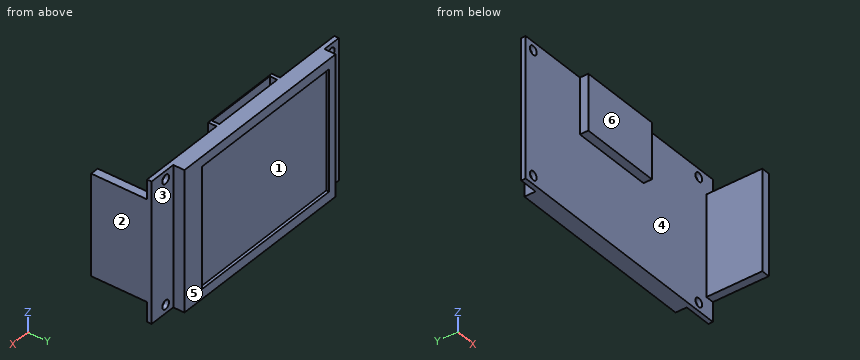
```python
from build123d import *

# Parameters (mm, degrees)
SKETCH1_W          = 86.3
SKETCH1_H          = 50.1
CIRCUIT_DEPTH      = 1.6
SKETCH2_R          = 1.57
SCREW_HOLES_DEPTH  = 50.919785657
SKETCH3_W          = 69.7
SKETCH3_H          = 50.1
LCD_DEPTH          = 4
SKETCH4_W          = 3
SKETCH4_H          = 36.1
PINS_DEPTH         = 20
SKETCH6_W          = 29.3
SKETCH6_H          = 20
SD_SLOT_DEPTH      = 3
SKETCH8_W          = 26.7
SKETCH8_H          = 2.65
CUT_EXTRUDE2_DEPTH = 5
SKETCH9_W          = 58.7
SKETCH9_H          = 43.1
CUT_EXTRUDE3_DEPTH = 1


with BuildPart() as part:
    # Sketch1 → CIRCUIT (new body)
    with BuildSketch(Plane(origin=(0, 0, 0), x_dir=(1, 0, 0), z_dir=(0, 1, 0))):
        Rectangle(SKETCH1_W, SKETCH1_H)
    extrude(amount=CIRCUIT_DEPTH)

    # Sketch2 → SCREW_HOLES (cut, through all)
    with BuildSketch(Plane(origin=(0, 1.6, 0), x_dir=(1, 0, 0), z_dir=(0, 1, 0))):
        with Locations(Location((-39.65, 22.05, 0), (0, 0, 270))):
            Circle(SKETCH2_R)
        with Locations(Location((-39.65, -22.05, 0), (0, 0, 270))):
            Circle(SKETCH2_R)
        with Locations(Location((36.65, 22.05, 0), (0, 0, 270))):
            Circle(SKETCH2_R)
        with Locations(Location((36.65, -22.05, 0), (0, 0, 270))):
            Circle(SKETCH2_R)
    extrude(amount=-SCREW_HOLES_DEPTH, mode=Mode.SUBTRACT)

    # Sketch3 → LCD (add)
    with BuildSketch(Plane(origin=(0, 1.6, 0), x_dir=(1, 0, 0), z_dir=(0, 1, 0))):
        with Locations((-1.7, 0)):
            Rectangle(SKETCH3_W, SKETCH3_H)
    extrude(amount=LCD_DEPTH)

    # Sketch4 → PINS (add)
    with BuildSketch(Plane.XZ):
        with Locations((41.65, 0)):
            Rectangle(SKETCH4_W, SKETCH4_H)
    extrude(amount=PINS_DEPTH)

    # Sketch6 → SD_SLOT (add)
    with BuildSketch(Plane.XZ):
        with Locations((-3.5, 15.05)):
            Rectangle(SKETCH6_W, SKETCH6_H)
    extrude(amount=SD_SLOT_DEPTH)

    # Sketch8 → Cut-Extrude2 (cut)
    with BuildSketch(Plane.XY.offset(25.05)):
        with Locations((-3.5, -1.325)):
            Rectangle(SKETCH8_W, SKETCH8_H)
    extrude(amount=-CUT_EXTRUDE2_DEPTH, mode=Mode.SUBTRACT)

    # Sketch9 → Cut-Extrude3 (cut)
    with BuildSketch(Plane(origin=(0, 5.6, 0), x_dir=(1, 0, 0), z_dir=(0, 1, 0))):
        with Locations((-4.2, 0)):
            Rectangle(SKETCH9_W, SKETCH9_H)
    extrude(amount=-CUT_EXTRUDE3_DEPTH, mode=Mode.SUBTRACT)


solid = part.part
```
For this review, take the finished solid that the model builds, in its own axes (mm). Face numbers are marked on the shaded views. A direction names the side the tool comes from. Coordinates: 2 decimals unless noted, no trailing zeros. Loops run counter-clockwise (first coordinate to the right, second up) from the corner with the lowest first, then second, coordinate; pieces in that order, holes last. Notation, with made-up numbers: (47, 2) - (97, 2) arc R23 ccw to (97, 15) - close; hole circle Ø5 at (22, 57). An arc over 180 degrees is marked (long way). Use one line per item in the form item = value. Start each with the question number.
1) Take a section at D-D (x = 20). State the section outline as (y, z) points, plus the area to 3 significant figures.
2) Take a section at B-B (x = -39.65). State the section outline as (y, z) points, plus the area to 3 significant figures.
3) For the marked faces 5 and 6, list the 3-axis set-ups (+Z, -Z, +X, -X, +Y, -Y) from which the entire face can be reached by the end or side of a thin tool; tool diameter is ignored.
4) For pin 1 (3.5 mm diameter, centred on x = -39.65, z = -22.05, fed in from +Y); pin 2 (4 mm diameter, centred on x = -5, z = 21.5, fed in from -Y); pin 3 (3.5 mm diameter, centred on x = 42.5, y = -9, fed in from +Z), all flat-tipped, find the tip position at first contact; note any pin that passes through.
5) Take a section at A-A (y = -1.75). State the section outline as (x, z) points, plus the area to 3 significant figures.
6) Take a section at C-C (z = -6). State the section outline as (x, y) points, plus the area to 3 significant figures.
7) Draft analysis for pull direction X (two halves, no side actions). For the marked faces 1, 2, 3 and 4, state which applies: released by +X, released by -X, zero draft, split by the parting line, or undercut.
8) To check wall thickness, follow probe 1 along X at (y, z) = (1.05, 22.05); probe 2 along Y at (x, z) = (-13, -5); probe 3 along X at (y, z) = (-16, 14). State the ranges of each line that lie inside material, in increasing order. Write a range as from..to.
From the geometry:
q1.outline = (0, -25.05) - (5.6, -25.05) - (5.6, -21.55) - (4.6, -21.55) - (4.6, 21.55) - (5.6, 21.55) - (5.6, 25.05) - (0, 25.05) - close
q1.area = 237 mm2
q2.outline = (0, -25.05) - (1.6, -25.05) - (1.6, -23.62) - (0, -23.62) - close; (0, -20.48) - (1.6, -20.48) - (1.6, 20.48) - (0, 20.48) - close; (0, 23.62) - (1.6, 23.62) - (1.6, 25.05) - (0, 25.05) - close
q2.area = 70.1 mm2
q3.face_5 = +Z, -Z, +X, -X, +Y
q3.face_6 = +Z, -Z, -X, -Y
q4.pin_1 = 1.6
q4.pin_2 = -3
q4.pin_3 = 18.05
q5.outline = (-18.15, 5.05) - (11.15, 5.05) - (11.15, 25.05) - (9.85, 25.05) - (9.85, 20.05) - (-16.85, 20.05) - (-16.85, 25.05) - (-18.15, 25.05) - close; (40.15, -18.05) - (43.15, -18.05) - (43.15, 18.05) - (40.15, 18.05) - close
q5.area = 561 mm2
q6.outline = (-43.15, 0) - (40.15, 0) - (40.15, -20) - (43.15, -20) - (43.15, 1.6) - (33.15, 1.6) - (33.15, 5.6) - (25.15, 5.6) - (25.15, 4.6) - (-33.55, 4.6) - (-33.55, 5.6) - (-36.55, 5.6) - (-36.55, 1.6) - (-43.15, 1.6) - close
q6.area = 418 mm2
q7.face_1 = undercut
q7.face_2 = released by +X
q7.face_3 = zero draft
q7.face_4 = undercut
q8.probe_1 = -43.15..-41.22, -38.08..35.08, 38.22..43.15
q8.probe_2 = 0..4.6
q8.probe_3 = 40.15..43.15
